Can you work these out from the drawing? Everything is in mm from the part's minimum corner. Coordinates: 2 decimals unless noted, no trailing zeros. Order: outer loops, then holes, each group sorted by start corner. A loop starts at its lowest first (then second) coordinate and runs counter-clockwise, first axis right, second up. Notation, with made-up numbers: (-37, 32.25) -> (-14, 32.25) arc R4 cw to (-14, 36.25) -> close; hole circle Ø5 at (71, 18.25). An arc over 180 degrees is marked (long way). Put each result on its own line as item: value. Start each with the question number.
Q1. Please list where these lines run through material, in increasing order: line 1 along Y through (x, z) = (4.5, 0.1) (1 decimal); line 2 along Y through (x, z) = (1.6, 0.25) (1 decimal); line 3 along X through (y, z) = (3, 0.4) (1 decimal).
Q2. We'd pull the mould along X, two halves only. Please class the marked faces 1, 2 and 3: +X half, -X half, draft (parallel to the pull), parting line (faces both ways), or undercut.
Q3. If we section it at A-A (x = 1.6): Please give me the cut outline in (y, z).
Q4. If we section it at C-C (x = 2.25): Please give me the cut outline in (y, z).
Q5. If we section it at B-B (y = 1.5): Please give me the cut outline in (x, z) (1 decimal).
Q6. If we section it at D-D (z = 0.15): Please give me the cut outline in (x, y) (1 decimal), and give its area (3 significant figures).
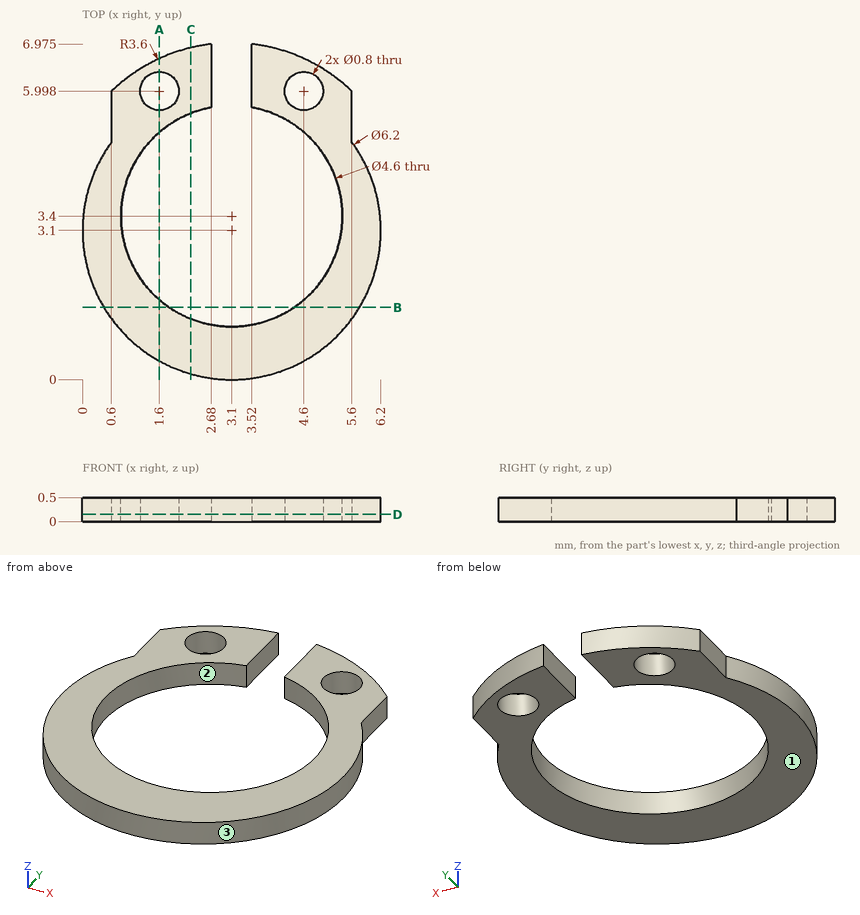
The answers:
1. line 1: 0.3 to 1.6, 5.2 to 5.6, 6.4 to 6.7
1. line 2: 0.4 to 1.7, 5.1 to 5.6, 6.4 to 6.7
1. line 3: 0 to 0.8, 5.4 to 6.2
2. face 1: draft
2. face 2: undercut
2. face 3: parting line
3. outline: (0.39, 0) -> (1.66, 0) -> (1.66, 0.5) -> (0.39, 0.5) -> close; (5.14, 0) -> (5.6, 0) -> (5.6, 0.5) -> (5.14, 0.5) -> close; (6.4, 0) -> (6.67, 0) -> (6.67, 0.5) -> (6.4, 0.5) -> close
4. outline: (0.12, 0) -> (1.26, 0) -> (1.26, 0.5) -> (0.12, 0.5) -> close; (5.54, 0) -> (6.9, 0) -> (6.9, 0.5) -> (5.54, 0.5) -> close
5. outline: (0.4, 0) -> (1.8, 0) -> (1.8, 0.5) -> (0.4, 0.5) -> close; (4.4, 0) -> (5.8, 0) -> (5.8, 0.5) -> (4.4, 0.5) -> close
6. outline: (0.6, 4.9) arc R3.1 ccw (long way) to (5.6, 4.9) -> (5.6, 6) arc R3.6 ccw to (3.5, 7) -> (3.5, 5.7) arc R2.3 cw (long way) to (2.7, 5.7) -> (2.7, 7) arc R3.6 ccw to (0.6, 6) -> close; hole circle Ø0.8 at (1.6, 6); hole circle Ø0.8 at (4.6, 6)
6. area: 15.8 mm^2
